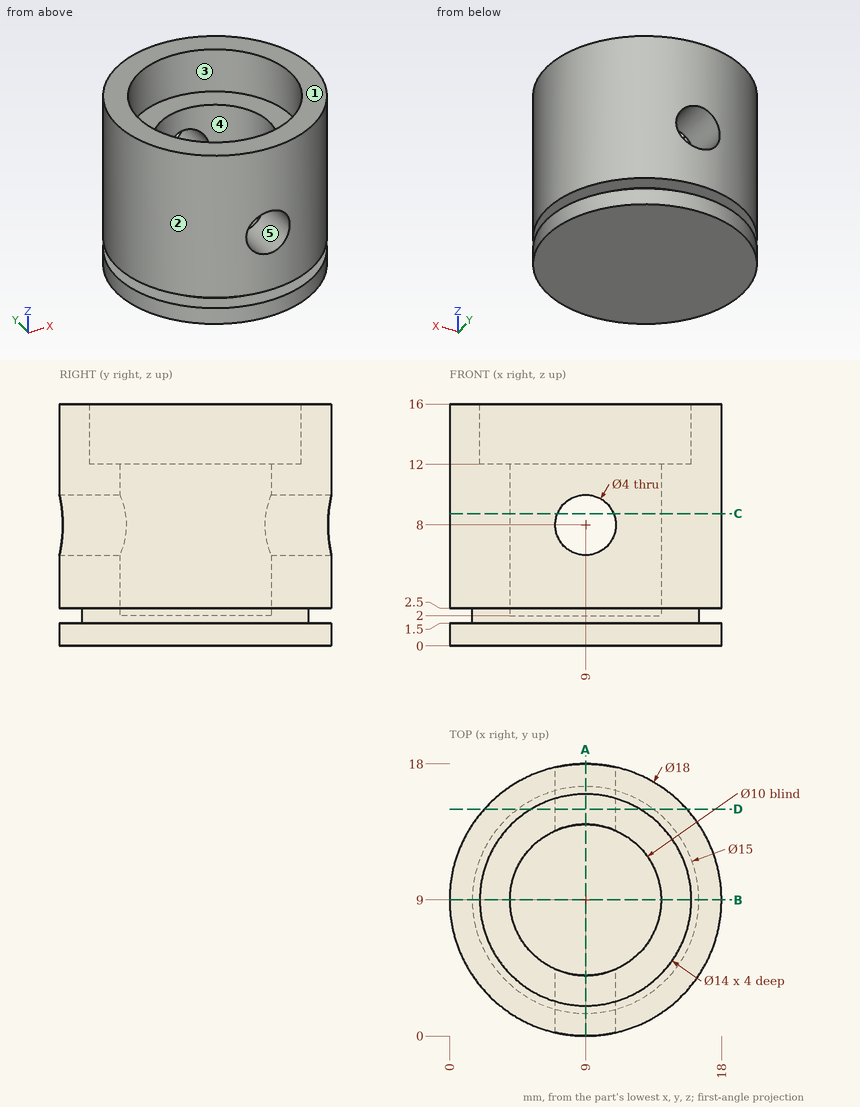
Job drawing, mm, ordinate dimensions from the low corner. One solid piece. A direction names the side the tool comes from. Round coordinates to 2 decimals unless told otherwise and drop trailing zeros. Order: outer loops, then holes, each group sorted by start corner. A loop starts at its lowest first (then second) coordinate and runs counter-clockwise, first axis right, second up. Notation, with made-up numbers: M 2,-28.75 L 23,-28.75 A12 ccw 23,-6.75 Z; hole C 17.25,5.25 d10. An arc over 180 degrees is marked long. Write each question's results on one line, items separated by ' | '. Start each with the question number.
(1) Saw through at B-B, the plane y = 9. Give the cut face in (x, z).
(2) Which spindle directions (+Z, -Z, +X, -X, +Y, -Y) get a long thin tool onto all of the face, cutting with end or side? Do the marked faces 4 and 5. Say none if no direction does.
(3) Drop flat-ended pins along their axis: pin 1 (2 mm diameter, centred on x = 4, z = 2.5, fed in from +Y); pin 2 (4 mm diameter, centred on x = 8, y = 9.5, fed in from +Z). Give the stop position or say it passes through.
(4) Probe probe 1 along Y at (x, z) = (9, 14.6); probe 2 along Z at (x, y) = (7.5, 1); probe 3 along Y at (x, z) = (9, 5.75). List the from-to ranges inside material, lowest first. Write a range as from..to.
(5) Saw through at A-A, the plane x = 9. Give the cut face in (y, z).
(6) Saw through at C-C, the plane z = 8.75. Give the cut face in (x, y).
(7) Two-plate mould, pull along Y, no slides. Class the marked faces 1, 2 and 3: pulls with the +Y half, pulls with the -Y half, needs draft (parallel to the pull), parting line crosses it, or undercut.
(8) Saw through at D-D, the plane y = 15. Give the cut face in (x, z), then the cut area to 3 significant figures.
Established:
1) outline: M 0,0 L 18,0 L 18,1.5 L 16.5,1.5 L 16.5,2.5 L 18,2.5 L 18,16 L 16,16 L 16,12 L 14,12 L 14,2 L 4,2 L 4,12 L 2,12 L 2,16 L 0,16 L 0,2.5 L 1.5,2.5 L 1.5,1.5 L 0,1.5 Z
2) face 4: +Z | face 5: +Y, -Y
3) pin 1: stops at y = 17.06 | pin 2: stops at z = 2
4) probe 1: y = 0..2, 16..18 | probe 2: z = 0..1.5, 2.5..6.68, 9.32..16 | probe 3: y = 0..4, 14..18
5) outline: M 0,0 L 18,0 L 18,1.5 L 16.5,1.5 L 16.5,2.5 L 18,2.5 L 18,6 L 14,6 L 14,2 L 4,2 L 4,6 L 0,6 L 0,2.5 L 1.5,2.5 L 1.5,1.5 L 0,1.5 Z; M 0,10 L 4,10 L 4,12 L 2,12 L 2,16 L 0,16 Z; M 14,10 L 18,10 L 18,16 L 16,16 L 16,12 L 14,12 Z
6) outline: M 7.15,0.19 L 7.15,4.36 A5 cw 7.15,13.64 L 7.15,17.81 A9 ccw Z; M 10.85,0.19 A9 ccw 10.85,17.81 L 10.85,13.64 A5 cw 10.85,4.36 Z
7) face 1: needs draft | face 2: parting line crosses it | face 3: undercut
8) outline: M 2.29,0 L 15.71,0 L 15.71,1.5 L 13.5,1.5 L 13.5,2.5 L 15.71,2.5 L 15.71,16 L 12.61,16 L 12.61,12 L 5.39,12 L 5.39,16 L 2.29,16 L 2.29,2.5 L 4.5,2.5 L 4.5,1.5 L 2.29,1.5 Z; hole C 9,8 d4 | area: 169 mm^2
